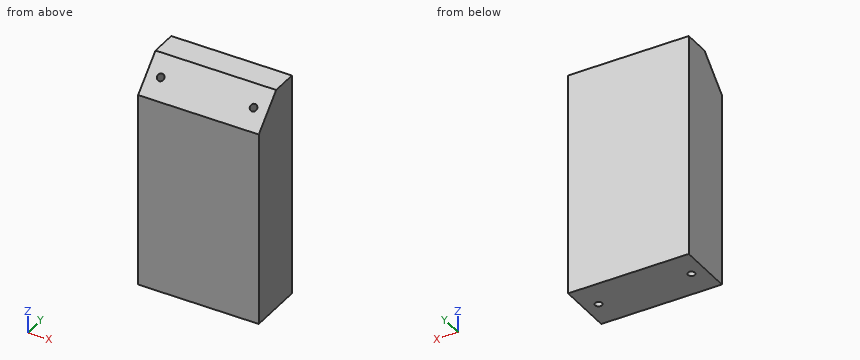
```python
from build123d import *

# Parameters (mm, degrees)
F0_W           = 82.55
F0_H           = 153.3652
F1_DEPTH       = 38.1
F2_SIZE2       = 20.0152
F2_SIZE        = 20.0152
F5_D           = 4.826
F5_DEPTH       = 12.7
F5_TIP         = 1.4498766737
F5_ON_F4_D     = 4.826
F5_ON_F4_DEPTH = 12.7
F5_ON_F4_TIP   = 1.4498766737


with BuildPart() as f1:
    # F0 (on Front) → F1 (new body)
    with BuildSketch(Plane.XZ):
        with Locations((41.275, 76.6826)):
            Rectangle(F0_W, F0_H)
    extrude(amount=F1_DEPTH)

    # F2
    f2_edges = [f1.edges().sort_by_distance(p)[0] for p in [
        (41.275, -38.1, 153.3652),
    ]]
    chamfer(f2_edges, length=F2_SIZE, length2=F2_SIZE2)

    # F5
    with Locations(Plane(origin=(0, -85.725, 85.725), x_dir=(1, 0, 0), z_dir=(0, -0.7071067812, 0.7071067812))):
        with Locations((9.525, 81.5048045548), (73.025, 81.5048045548)):
            Hole(F5_D / 2, depth=F5_DEPTH)
            with Locations((0, 0, -(F5_DEPTH + F5_TIP / 2))):  # 118° drill point
                Cone(0, F5_D / 2, F5_TIP, mode=Mode.SUBTRACT)

    # F5 on F4
    with Locations(Plane(origin=(0, 0, 0), x_dir=(1, 0, 0), z_dir=(0, 0, -1))):
        with Locations((9.525, 19.05), (73.025, 19.05)):
            Hole(F5_ON_F4_D / 2, depth=F5_ON_F4_DEPTH)
            with Locations((0, 0, -(F5_ON_F4_DEPTH + F5_ON_F4_TIP / 2))):  # 118° drill point
                Cone(0, F5_ON_F4_D / 2, F5_ON_F4_TIP, mode=Mode.SUBTRACT)


solid = f1.part
```
Here's how the part is built. I have some questions about the finished solid (model axes, mm). Give positions to 0.01 mm unless a question says otherwise; leave off trailing zeros. Write each loop counter-clockwise with the first axis right and the second up, starting at its lowest first coordinate (ties: lowest second). Pieces come first, ordered by that corner, then holes.
(1) If I drill on L1, parallel to X at y = -19.05, z = 4.25; L2, parallel to Y at x = 71.5, z = 11; L3, parallel to Z at x = 55.5, y = -24, over which ranges is the centre line in solid material (lowest first)?
Output values:
L1: x = 0 to 7.11, 11.94 to 70.61, 75.44 to 82.55
L2: y = -38.1 to -20.92, -17.18 to 0
L3: z = 0 to 147.45
(2) Imagine slicing it at A-A, the plane x = 56.5. Write out the boundary of the cut face in (y, z), and give its area (3 significant figures).
Output values:
outline: (-38.1, 0) - (0, 0) - (0, 153.37) - (-18.08, 153.37) - (-38.1, 133.35) - close
area: 5,640 mm2
(3) Will this pin go through, and if not, where does the flat tip stop? pin 1 (2 mm diameter, centred on x = 62.5, y = -33, fed in from +Z).
Output values:
pin 1: stops at z = 139.45
